Autodesk Inventor part; units mm, degrees
ref_plane "YZ Plane" through (0, 0, 0) normal (1, 0, 0) x (0, 1, 0)
ref_plane "XZ Plane" through (0, 0, 0) normal (0, 1, 0) x (-1, 0, 0)
ref_plane "XY Plane" through (0, 0, 0) normal (0, 0, 1) x (1, 0, 0)
sketch "Sketch1" plane through (0, 0, 0) normal (1, 0, 0) x (0, 1, 0)
  circle A0 centre (0, 0) radius 1.5
  line L0 (-30.1, 0) -> (30.1, 0)
  line L1 (1.118, -1) -> (-1.118, -1)
  circle A1 centre (0, 0) radius 9
  circle A2 centre (0, 0) radius 21.5
  circle A3 centre (0, 0) radius 18.5
  dimension "d0" = 3
  dimension "d1" = 1
  dimension "d3" = 43
  dimension "d4" = 3
  dimension "d6" = 18
extrude "Extrusion1" add sketch "Sketch1" along normal blind 5 contours L1 A0 | A0 L0 A1 | L0 A1 A0
sketch "Sketch3" plane through (0, 0, 0) normal (0, 0, 1) x (1, 0, 0)
  line L0 (0, 9) -> (5, 9)
  line L1 (-1, 0) -> (6, 0)
  circle A0 centre (1.7822, 7.75) radius 1.25
  line L2 (0.5662, 7.4607) -> (0.2, 9)
  line L3 (0, 9) -> (5, 9)
  line L4 (0, 10) -> (5, 10)
  line L5 (0, 9) -> (5, 9)
  line L6 (4.8, 9) -> (2.6661, 6.8661)
  line L7 (4.8, 9) -> (4.8, 9)
  line L8 (4.8, 9) -> (5, 9)
  line L9 (5, -9) -> (5, 9)
  line L10 (5, 9) -> (5, 9)
  line L11 (0, -9) -> (0, 9)
  line L12 (0.2, 9) -> (0, 9)
  point P0 (0, 0)
  point P1 (1.7822, 9)
  point P2 (4.8, 9)
  dimension "d20" = 2.5
  dimension "d26" = 45
  dimension "d28" = 0.2
revolve "Revolution1" cut sketch "Sketch3" angle 360 about axis through (-10, 0, 0) along (-1, 0, 0) contours L0 A0 L2 | L0 L6 A0 | A0
sketch "Sketch2" plane through (0, 0, 0) normal (-1, 0, 0) x (0, 0, 1)
  circle A0 centre (0, 0) radius 21.5
  circle A1 centre (0, 0) radius 19.9
  circle A2 centre (0, 0) radius 9
  line L0 (-1, 1.118) -> (-1, -1.118)
  arc A3 (-1, -1.118) -> (-1, 1.118) centre (0, 0) ccw
  line L1 (3.2444, 19.6337) -> (6.4888, 14.0143)
  line L2 (6.4888, 14.0143) -> (3.2444, 8.3949)
  line L3 (3.2444, 8.3949) -> (-3.2444, 8.3949)
  line L4 (-3.2444, 8.3949) -> (-6.4888, 14.0143)
  line L5 (-6.4888, 14.0143) -> (-3.2444, 19.6337)
  line L6 (-3.2444, 19.6337) -> (3.2444, 19.6337)
  line L7 (0, -30.1) -> (0, 30.1)
  line L8 (-2.7825, 18.8337) -> (-5.565, 14.0143)
  line L9 (-5.565, 14.0143) -> (-2.7825, 9.1949)
  line L10 (-2.7825, 9.1949) -> (2.7825, 9.1949)
  line L11 (2.7825, 9.1949) -> (5.565, 14.0143)
  line L12 (5.565, 14.0143) -> (2.7825, 18.8337)
  line L13 (2.7825, 18.8337) -> (-2.7825, 18.8337)
  line L14 (-17.6702, 9.1528) -> (-11.3233, 10.5018)
  line L15 (-19.6754, 2.9816) -> (-17.6702, 9.1528)
  line L16 (-15.3335, -1.8405) -> (-19.6754, 2.9816)
  line L17 (-8.9866, -0.4914) -> (-15.3335, -1.8405)
  line L18 (-15.0481, -0.962) -> (-9.6047, 0.1951)
  line L19 (-9.6047, 0.1951) -> (-7.885, 5.4877)
  line L20 (-7.885, 5.4877) -> (-11.6087, 9.6233)
  line L21 (-11.3233, 10.5018) -> (-6.9814, 5.6798)
  line L22 (-6.9814, 5.6798) -> (-8.9866, -0.4914)
  line L23 (-11.6087, 9.6233) -> (-17.0521, 8.4663)
  line L24 (-17.0521, 8.4663) -> (-18.7718, 3.1736)
  line L25 (-18.7718, 3.1736) -> (-15.0481, -0.962)
  line L26 (-14.1652, -13.977) -> (-13.4869, -7.5238)
  line L27 (-8.9157, -17.791) -> (-14.1652, -13.977)
  line L28 (-2.9879, -15.1518) -> (-8.9157, -17.791)
  line L29 (-2.3096, -8.6986) -> (-2.9879, -15.1518)
  line L30 (-3.7352, -14.6088) -> (-3.1535, -9.0743)
  line L31 (-3.1535, -9.0743) -> (-7.6557, -5.8033)
  line L32 (-7.6557, -5.8033) -> (-12.7396, -8.0668)
  line L33 (-13.4869, -7.5238) -> (-7.5591, -4.8846)
  line L34 (-7.5591, -4.8846) -> (-2.3096, -8.6986)
  line L35 (-12.7396, -8.0668) -> (-13.3213, -13.6013)
  line L36 (-13.3213, -13.6013) -> (-8.8191, -16.8723)
  line L37 (-8.8191, -16.8723) -> (-3.7352, -14.6088)
  line L38 (8.9157, -17.791) -> (2.9879, -15.1518)
  line L39 (14.1652, -13.977) -> (8.9157, -17.791)
  line L40 (13.4869, -7.5238) -> (14.1652, -13.977)
  line L41 (7.5591, -4.8846) -> (13.4869, -7.5238)
  line L42 (12.7396, -8.0668) -> (7.6557, -5.8033)
  line L43 (7.6557, -5.8033) -> (3.1535, -9.0743)
  line L44 (3.1535, -9.0743) -> (3.7352, -14.6088)
  line L45 (2.9879, -15.1518) -> (2.3096, -8.6986)
  line L46 (2.3096, -8.6986) -> (7.5591, -4.8846)
  line L47 (3.7352, -14.6088) -> (8.8191, -16.8723)
  line L48 (8.8191, -16.8723) -> (13.3213, -13.6013)
  line L49 (13.3213, -13.6013) -> (12.7396, -8.0668)
  line L50 (19.6754, 2.9816) -> (15.3335, -1.8405)
  line L51 (17.6702, 9.1528) -> (19.6754, 2.9816)
  line L52 (11.3233, 10.5018) -> (17.6702, 9.1528)
  line L53 (6.9814, 5.6798) -> (11.3233, 10.5018)
  line L54 (11.6087, 9.6233) -> (7.885, 5.4877)
  line L55 (7.885, 5.4877) -> (9.6047, 0.1951)
  line L56 (9.6047, 0.1951) -> (15.0481, -0.962)
  line L57 (15.3335, -1.8405) -> (8.9866, -0.4914)
  line L58 (8.9866, -0.4914) -> (6.9814, 5.6798)
  line L59 (15.0481, -0.962) -> (18.7718, 3.1736)
  line L60 (18.7718, 3.1736) -> (17.0521, 8.4663)
  line L61 (17.0521, 8.4663) -> (11.6087, 9.6233)
  point P0 (0, 14.0143)
  point P1 (3.2444, 8.3949)
  point P2 (-17.6702, 9.1528)
  point P3 (-6.9814, 5.6798)
  point P4 (-19.6754, 2.9816)
  point P5 (-8.9866, -0.4914)
  point P6 (-7.5591, -4.8846)
  point P7 (-14.1652, -13.977)
  point P8 (-8.9157, -17.791)
  point P9 (-2.3096, -8.6986)
  point P10 (2.3096, -8.6986)
  point P11 (8.9157, -17.791)
  point P12 (14.1652, -13.977)
  point P13 (7.5591, -4.8846)
  point P14 (8.9866, -0.4914)
  point P15 (19.6754, 2.9816)
  point P16 (17.6702, 9.1528)
  point P17 (6.9814, 5.6798)
  dimension "d9" = 43
  dimension "d10" = 1.6
  dimension "d11" = 0.8
  dimension "d31" = 360
extrude "Extrusion2" add sketch "Sketch2" along normal blind 7 contours A0 L7 A1 | L7 A1 A0 | L7 L6 A1 | A1 L6 L7 | L1 L2 A2 L7 L10 L11 L12 L13 L6 | L6 L7 L13 L8 L9 L10 A2 L4 L5 | A1 L27 | L27 L26 L33 A2 L29 L28 | L39 A1 | L38 L45 A2 L41 L40 L39 | L7 A3 L3 A2 L58 L46 | A2 L34 L22 L3 L7 A3 L0 | A1 L51 | L51 L50 L57 A2 L53 L52 | L15 A1 | L14 L21 A2 L17 L16 L15 | A2 L34 | L46 A2 | L3 L7 A2 | A2 L7 L3 | A2 L58 | L22 A2
sketch "Sketch4" plane through (0, 0, 0) normal (0, 0, 1) x (1, 0, 0)
  line L0 (0, 21.5) -> (-7, 21.5)
  line L1 (-7, 21.5) -> (-7, -21.5)
  arc A0 (0, 21.5) -> (-7, 21.5) centre (-3.5, 15.875) ccw
  line L2 (-8.4, 0) -> (1.4, 0)
  point P0 (0, 0)
  point P1 (-3.5, 22.5)
  dimension "d24" = 1
revolve "Revolution2" add sketch "Sketch4" angle 360 about axis through (-10, 0, 0) along (1, 0, 0)
equation "\"d6\" = WheelGrooveDia"
equation "\"d7\" = WheelGrooveWidth"
equation "\"d20\" = WheelPulleyDia"
equation "\"d9\" = WheelDia - 2 * Roundedness"
equation "\"d16\" = WheelWidth"
equation "\"Roundedness\" = 1"
properties part number "PulleyedWheelV1" material "H TPU"
CAD build for the part. Positions are in the model's coordinates, mm. A direction names the side the tool comes from. Round coordinates to 2 decimals unless told otherwise and drop trailing zeros. Order: outer loops, then holes, each group sorted by start corner. A loop starts at its lowest first (then second) coordinate and runs counter-clockwise, first axis right, second up. Notation, with made-up numbers: (41, 14) - (70, 14) arc R16 ccw to (70, 40) - close; hole circle Ø1 at (55, 36). An arc over 180 degrees is marked (long way). Answer in a Markdown table with one row per item. Add a question column.
(1) Drop flat-ended pins along their axis: pin 1 Ø5 at (x, z) = (3.5, 9) entering from -Y; pin 2 Ø1.8 at (x, y) = (0, -0.5) entering from +Z; pin 3 Ø2 at (x, z) = (-4.5, -1.5) entering from -Y. Give the stop position or say it passes through.
(2) Band-saw the part on B-B on x = -5.75. Count the separate pieces of the cut face and the enclosed holes in it, and give its area (3 significant figures).
(3) Band-saw the part on A-A on z = 0. List the corners of the cut face in (x, y) (3 decimals).
(4) 3-axis set-ups, long thin cutter, end or side, ignore diameter. For faces 1 (the face through (5, 0, -2)), 2 (the face through (-3.451, -10.873, 13.035)): which of +Z, -Z, +X, -X, +Y, -Y reach the whole face in a straight line?
(5) Mould opens along Y. For faces 3 (the face through (-3.451, -0.375, 12.288)), 4 (the face through (-3.451, 8.057, 9.122)), 5 (the face through (-7, 2, 0)) say: +Y half, -Y half, draft (parallel to the pull), parting line (faces both ways), or undercut.
(6) Probe L1, parallel to Y at x = -1.5, z = 0; L2, parallel to Y at x = -5, z = 10.5; L3, parallel to Z at x = -2.5, y = 4. List the from-to ranges inside material, lowest first. Write a range as [from, to].
Data:
| question | item | result |
|---|---|---|
| 1 | pin 1 | stops at y = -5.82 |
| 1 | pin 2 | stops at z = 21.96 |
| 1 | pin 3 | stops at y = -22.48 |
| 2 | separate pieces | 1 |
| 2 | enclosed holes | 11 |
| 2 | area | 677 mm^2 |
| 3 | outline | (-7, -21.5) arc R6.625 ccw to (0, -21.5) - (0, -19.9) - (-7, -19.9) - close; (-7, -9) - (0.2, -9) - (0.566, -7.461) arc R1.25 cw to (2.666, -6.866) - (4.8, -9) - (5, -9) - (5, -1.5) - (-7, -1.5) - close; (-7, 1.5) - (5, 1.5) - (5, 9) - (4.8, 9) - (2.666, 6.866) arc R1.25 cw to (0.566, 7.461) - (0.2, 9) - (0, 9) - (0, 9.195) - (-7, 9.195) - close; (-7, 18.834) - (0, 18.834) - (0, 21.5) arc R6.625 ccw to (-7, 21.5) - close |
| 4 | face 1 | +Z, -Z, +X, +Y, -Y |
| 4 | face 2 | +X, -X |
| 5 | face 3 | undercut |
| 5 | face 4 | undercut |
| 5 | face 5 | draft |
| 6 | L1 | y = [-22.19, -19.9], [-9, -1.5], [1.5, 9.19], [18.83, 22.19] |
| 6 | L2 | y = [-19.71, -15.65], [-7.07, -6.19], [-0.81, 0], [8.39, 9.59], [16.9, 19.71] |
| 6 | L3 | z = [-22.06, -18.5], [-8.37, 8.37], [18.5, 22.06] |
